from build123d import *

# Parameters (mm, degrees)
F1_DEPTH = 7
F2_R     = 0.5
F3_R     = 4
F4_DEPTH = 100
F5_SIZE  = 1


with BuildPart() as f1:
    # F0 (on Top) → F1 (new body)
    with BuildSketch(Plane.XY):
        Polygon((1.807803, 7.284585), (-5.404734, 5.207896), (-7.212537, -2.076689), (-1.807803, -7.284585), (5.404734, -5.207896), (7.212537, 2.076689), align=None)
    extrude(amount=F1_DEPTH)

    # F2
    f2_edges = [f1.edges().sort_by_distance(p)[0] for p in [
        (-4.51017, -4.680637, 7),
        (1.798465, -6.246241, 7),
        (4.51017, 4.680637, 7),
        (-1.798465, 6.246241, 7),
        (-6.308636, 1.565604, 7),
        (6.308636, -1.565604, 7),
    ]]
    fillet(f2_edges, radius=F2_R)

    # F3 (on face) → F4 (join)
    with BuildSketch(Plane(origin=(0, 0, 0), x_dir=(1, 0, 0), z_dir=(0, 0, -1))):
        Circle(F3_R)
    extrude(amount=F4_DEPTH)

    # F5
    f5_edges = [f1.edges().sort_by_distance(p)[0] for p in [
        (-4, 0, -100),
    ]]
    chamfer(f5_edges, length=F5_SIZE)


solid = f1.part
Check sheet for the modelled part. Datum: model origin and axes. Units: mm. A direction names the side the tool comes from. Give positions to 0.01 mm unless a question says otherwise; leave off trailing zeros. Write each loop counter-clockwise with the first axis right and the second up, starting at its lowest first coordinate (ties: lowest second). Pieces come first, ordered by that corner, then holes. Notation, with made-up numbers: (22, -34) -> (75, -34) arc R34 cw to (75, 0) -> close; hole circle Ø1 at (-13, -33.5). An arc over 180 degrees is marked (long way). One line per item, written item: value. Start each with the question number.
Item 1: Gauge pin test, flat ends, axial feed: pin 1 (4 mm diameter, centred on y = -4.5, z = -16.5, fed in from -X); pin 2 (3 mm diameter, centred on x = -3.5, z = -80, fed in from -Y); pin 3 (6 mm diameter, centred on y = -2, z = -17.5, fed in from -X). Record the tip position at first contact, or that the pin passes through.
Item 2: Tool access check on faces 1 (the flat face through (-1.75, 6.26, 3.2)), 2 (the flat face through (3, -3, 0)). Record the directions out of +Z, -Z, +X, -X, +Y, -Y that give a thin tool (end or side, any length) a straight path to the whole face; none if there is none.
Item 3: Material ranges on probe 1 along Y at (x, z) = (-0.25, -72); probe 2 along Y at (x, z) = (-3.5, -85.5); probe 3 along Z at (x, y) = (-0.25, -4.25), recorded low to high. Write a range as from..to.
Item 4: Section check A-A on z = -89.5. Record the cut outline in (x, y), then the cut area to 3 significant figures.
Results list:
1. pin 1: x = -3.12
1. pin 2: y = -3.46
1. pin 3: x = -4
2. face 1: +Z, -Z, -X, +Y
2. face 2: -Z
3. probe 1: -3.99..3.99
3. probe 2: -1.94..1.94
3. probe 3: 0..7
4. outline: circle Ø8 at (0, 0)
4. area: 50.3 mm²
